Geometry: final body of the model. Coordinates: model frame, mm. Face numbers are marked on the shaded views. A direction names the side the tool comes from. Round coordinates to 2 decimals unless told otherwise and drop trailing zeros. Write each loop counter-clockwise with the first axis right and the second up, starting at its lowest first coordinate (ties: lowest second). Pieces come first, ordered by that corner, then holes. Notation, with made-up numbers: (-27.5, -35) -> (-9.5, -35) arc R24 ccw to (-9.5, -22) -> close; hole circle Ø4 at (58.25, 32.5). An arc over 180 degrees is marked (long way). Use one line per item in the form item = value. Start each with the question number.
1. Cut plane D-D, the plane x = 33.5. State how many separate pieces and enclosed holes the cut face has, plus the area to 3 significant figures.
2. Cut plane B-B, the plane y = 26. Return the cut outline in (x, z), plus the area to 3 significant figures.
3. Cut plane C-C, the plane z = -3.75. Return the cut outline in (x, y), plus the area to 3 significant figures.
4. Pin query (flat end, axial travel): pin 1 Ø4 at (x, z) = (-35, 1) entering from -Y; pin 2 Ø3 at (y, z) = (3, 2.5) entering from -X; pin 3 Ø5 at (x, z) = (-53, 1) entering from -Y. Return the tip coordinate at first contact, or that it passes through.
5. Line query: L1, parallel to Y at x = -50.5, z = 3.5; L2, parallel to Z at x = 28, y = -25; L3, parallel to Z at x = -22, y = -3. Output: solid intervals per line, ascending.
6. Draft query along Y for the marked faces 4, 5, 6 and 7. Return one class per face: pulls with the +Y half, pulls with the -Y half, needs draft (parallel to the pull), parting line crosses it, or undercut.
7. Reachability of the marked faces 1, 2 and 3 from +Z, -Z, +X, -X, +Y, -Y: full face, straight path, thin tool, end or side. Return the list, or none.
8. Cut plane A-A, the plane x = -37. Return the cut outline in (y, z), plus the area to 3 significant figures.
```python
from build123d import *

# Parameters (mm, degrees)
BOSS_EXTRUDE1_DEPTH         = 5
SKETCH2_R                   = 2.5
CUT_EXTRUDE1_DEPTH          = 84.719770664
SKETCH3_R                   = 2.5
CUT_EXTRUDE2_DEPTH          = 84.719770664
FILLET1_R                   = 5
Y_KSEKLIK_EKSTR_ZYON1_DEPTH = 20


with BuildPart() as part:
    # Sketch1 → Boss-Extrude1 (new, symmetric)
    with BuildSketch(Plane.XY):
        Polygon((-42.5, 4.25), (-38, 4.25), (-38, 2), (-33, 2), (-33, -2), (-38, -2), (-38, -4.25), (-42.5, -4.25), (-42.5, -2), (-46, -2), (-46, -6), (-56, -6), (-56, -16), (-46, -16), (-46, -20), (22, -20), (22, -30), (46, -30), (46, -20), (46, -16), (46, -6), (46, -2), (46, 2), (46, 6), (46, 16), (46, 20), (46, 30), (22, 30), (22, 20), (-46, 20), (-46, 16), (-56, 16), (-56, 6), (-46, 6), (-46, 2), (-42.5, 2), align=None)
    extrude(amount=BOSS_EXTRUDE1_DEPTH, both=True)

    # Sketch2 → Cut-Extrude1 (cut, through all)
    with BuildSketch(Plane.ZY.offset(-22)):
        with Locations(Location((0, -25, 0), (0, 0, 270))):
            Circle(SKETCH2_R)
    extrude(amount=-CUT_EXTRUDE1_DEPTH, mode=Mode.SUBTRACT)

    # Sketch3 → Cut-Extrude2 (cut, through all)
    with BuildSketch(Plane.ZY.offset(-22)):
        with Locations((0, 25)):
            Circle(SKETCH3_R)
    extrude(amount=-CUT_EXTRUDE2_DEPTH, mode=Mode.SUBTRACT)

    # Fillet1
    fillet1_edges = [part.edges().sort_by_distance(p)[0] for p in [
        (34, -30, 5),
        (34, -30, -5),
        (34, 30, 5),
        (34, 30, -5),
    ]]
    fillet(fillet1_edges, radius=FILLET1_R - 0.0001)  # a hair under: the kernel refuses the full size

    # Çizim2 → Yükseklik-Ekstrüzyon1 (add, symmetric)
    with BuildSketch(Plane(origin=(0, 0, 0), x_dir=(1, 0, 0), z_dir=(0, 1, 0))):
        with BuildLine():
            Line((46, 5), (-4, 5))
            add(Edge.make_bspline(
                [(-4, 5), (21.025086812, 6.697636519), (46, 9)],
                knots=[0, 0, 0, 1, 1, 1], degree=2))
            Line((46, 9), (46, 5))
        make_face()
    y_kseklik_ekstr_zyon1 = extrude(amount=Y_KSEKLIK_EKSTR_ZYON1_DEPTH, both=True)

    # Mirror1: Yükseklik-Ekstrüzyon1 across plane
    add(y_kseklik_ekstr_zyon1.mirror(Plane.XY))


solid = part.part
```
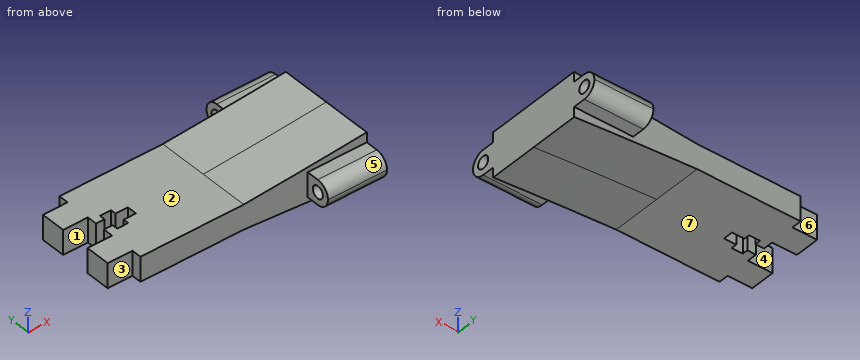
Outcome:
q1.separate_pieces = 1
q1.enclosed_holes = 2
q1.area = 770 mm^2
q2.outline = (22, -4.9) -> (46, -4.9) -> (46, -2.29) -> (22, -2.29) -> close; (22, 2.29) -> (46, 2.29) -> (46, 4.9) -> (22, 4.9) -> close
q2.area = 125 mm^2
q3.outline = (-56, -16) -> (-46, -16) -> (-46, -20) -> (22, -20) -> (22, -28.31) -> (46, -28.31) -> (46, 28.31) -> (22, 28.31) -> (22, 20) -> (-46, 20) -> (-46, 16) -> (-56, 16) -> (-56, 6) -> (-46, 6) -> (-46, 2) -> (-42.5, 2) -> (-42.5, 4.25) -> (-38, 4.25) -> (-38, 2) -> (-33, 2) -> (-33, -2) -> (-38, -2) -> (-38, -4.25) -> (-42.5, -4.25) -> (-42.5, -2) -> (-46, -2) -> (-46, -6) -> (-56, -6) -> close
q3.area = 4,210 mm^2
q4.pin_1 = -20
q4.pin_2 = -46
q4.pin_3 = -16
q5.L1 = -16 to -6, 6 to 16
q5.L2 = -5 to -2.5, 2.5 to 5
q5.L3 = -5 to 5
q6.face_4 = undercut
q6.face_5 = pulls with the -Y half
q6.face_6 = pulls with the +Y half
q6.face_7 = needs draft
q7.face_1 = +Z, -Z, -X
q7.face_2 = +Z, -X, +Y, -Y
q7.face_3 = +Z, -Z, -X, -Y
q8.outline = (-20, -5) -> (-2, -5) -> (-2, 5) -> (-20, 5) -> close; (2, -5) -> (20, -5) -> (20, 5) -> (2, 5) -> close
q8.area = 360 mm^2
